Drawing for the job (mm, zero at the part's lowest x, y, z). A direction names the side the tool comes from. Give positions to 0.01 mm unless a question says otherwise; leave off trailing zeros. Write each loop counter-clockwise with the first axis right and the second up, starting at its lowest first coordinate (ties: lowest second). Pieces come first, ordered by that corner, then holes.
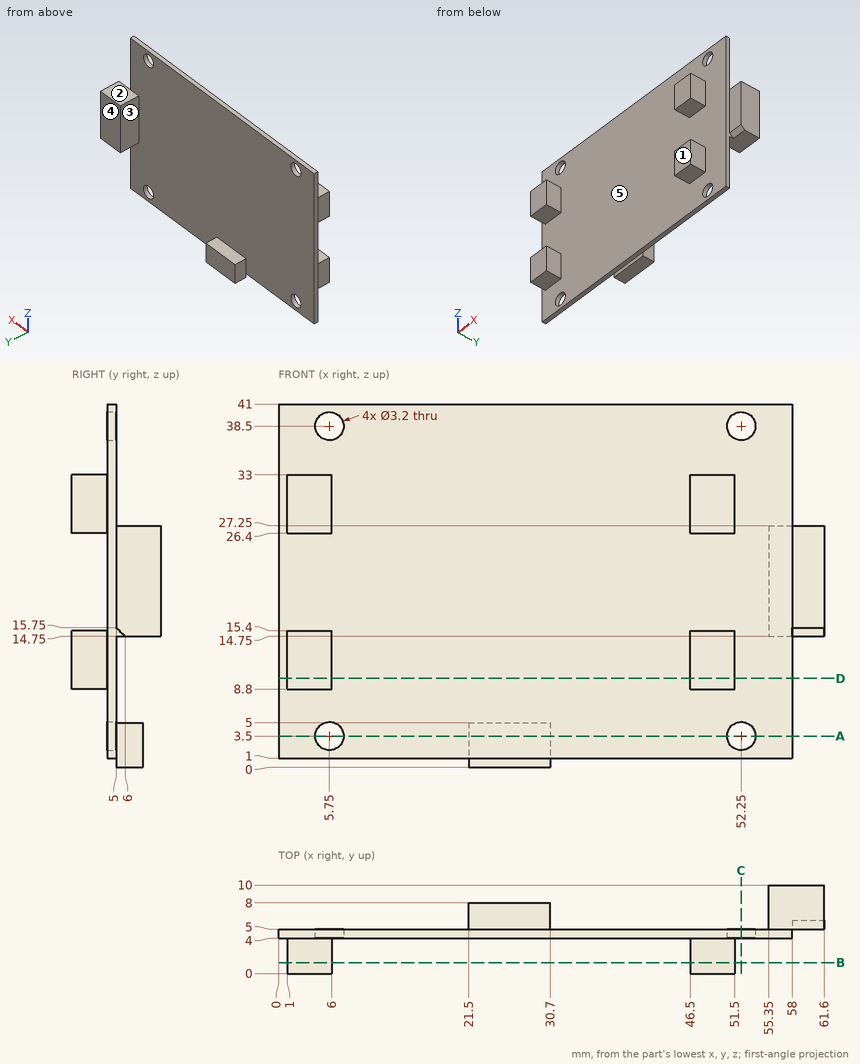
1. Slice it at A-A, the plane z = 3.5. Write the cut outline in (x, y).
Calculated:
outline: (0, 4) - (4.15, 4) - (4.15, 5) - (0, 5) - close; (7.35, 4) - (50.65, 4) - (50.65, 5) - (30.7, 5) - (30.7, 8) - (21.5, 8) - (21.5, 5) - (7.35, 5) - close; (53.85, 4) - (58, 4) - (58, 5) - (53.85, 5) - close
2. Pin check, flat tips, straight feed: P1, Ø1.5, axis at y = 6.5, z = 3.5, coming from the +X side; P2, Ø2, axis at y = 8.5, z = 14.5, coming from the -X side; P3, Ø3, axis at x = 21, y = 4, coming from the -Z side; P4, Ø1.1, axis at x = 28, z = 0.5, coming from the -Y side. Stop position of each tip, or through.
Calculated:
P1: stops at x = 30.7
P2: stops at x = 55.35
P3: stops at z = 0
P4: stops at y = 4
3. Probe probe 1 along X at (y, z) = (4.4, 38.5); probe 2 along Z at (x, y) = (52.25, 4.5); probe 3 along Z at (x, y) = (49, 3). List the from-to ranges inside material, lowest first.
Calculated:
probe 1: x = 0 to 4.15, 7.35 to 50.65, 53.85 to 58
probe 2: z = 1 to 1.9, 5.1 to 36.9, 40.1 to 41
probe 3: z = 8.8 to 15.4, 26.4 to 33
4. Slice it at D-D, the plane z = 10. Write the cut outline in (x, y), and give its area (3 significant figures).
Calculated:
outline: (0, 4) - (1, 4) - (1, 0) - (6, 0) - (6, 4) - (46.5, 4) - (46.5, 0) - (51.5, 0) - (51.5, 4) - (58, 4) - (58, 5) - (0, 5) - close
area: 98.0 mm2
5. Which spindle directions (+Z, -Z, +X, -X, +Y, -Y) get a long thin tool onto all of the face, cutting with end or side? Do the marked faces 1 and 2. Say none if no direction does.
Calculated:
face 1: +Z, -Z, +X, -X, -Y
face 2: +Z, +X, -X, +Y
6. Slice it at B-B, the plane y = 1.25. Write the cut outline in (x, z), and give its area (3 significant figures).
Calculated:
outline: (1, 8.8) - (6, 8.8) - (6, 15.4) - (1, 15.4) - close; (1, 26.4) - (6, 26.4) - (6, 33) - (1, 33) - close; (46.5, 8.8) - (51.5, 8.8) - (51.5, 15.4) - (46.5, 15.4) - close; (46.5, 26.4) - (51.5, 26.4) - (51.5, 33) - (46.5, 33) - close
area: 132 mm2
7. Slice it at C-C, the plane x = 52.25. Write the cut outline in (y, z).
Calculated:
outline: (4, 1) - (5, 1) - (5, 1.9) - (4, 1.9) - close; (4, 5.1) - (5, 5.1) - (5, 36.9) - (4, 36.9) - close; (4, 40.1) - (5, 40.1) - (5, 41) - (4, 41) - close
8. Pull direction X, two halves, no side cores. Call the marked faces 3, 4 and 5: +X half, -X half, draft (parallel to the pull), parting line (faces both ways), or undercut.
Calculated:
face 3: -X half
face 4: draft
face 5: undercut
